```python
from build123d import *

# Parameters (mm, degrees)
SKETCH1_W           = 129
SKETCH1_H           = 74
BOSS_EXTRUDE1_DEPTH = 39
SKETCH2_R           = 1.5
CUT_EXTRUDE1_DEPTH  = 10
SKETCH4_W           = 129
SKETCH4_H           = 24
CUT_EXTRUDE3_DEPTH  = 100


with BuildPart() as part:
    # Sketch1 → Boss-Extrude1 (new body)
    with BuildSketch(Plane.XY):
        with Locations((64.5, 37)):
            Rectangle(SKETCH1_W, SKETCH1_H)
    extrude(amount=-BOSS_EXTRUDE1_DEPTH)

    # Sketch2 → Cut-Extrude1 (cut)
    with BuildSketch(Plane(origin=(0, 0, -39), x_dir=(-1, 0, 0), z_dir=(0, 0, -1))):
        with Locations((-50.3, 37)):
            Circle(SKETCH2_R)
        with Locations((-50.3, 55.35)):
            Circle(SKETCH2_R)
        with Locations((-50.3, 18.65)):
            Circle(SKETCH2_R)
        with Locations((-20.3, 55.35)):
            Circle(SKETCH2_R)
        with Locations((-20.3, 37)):
            Circle(SKETCH2_R)
        with Locations((-20.3, 18.65)):
            Circle(SKETCH2_R)
        with Locations((-112.7, 37)):
            Circle(SKETCH2_R)
        with Locations((-112.7, 53)):
            Circle(SKETCH2_R)
        with Locations((-110.1, 58.75)):
            Circle(SKETCH2_R)
        with Locations((-110.1, 46.75)):
            Circle(SKETCH2_R)
        with Locations((-110.1, 15.25)):
            Circle(SKETCH2_R)
        with Locations((-110.1, 27.25)):
            Circle(SKETCH2_R)
    extrude(amount=-CUT_EXTRUDE1_DEPTH, mode=Mode.SUBTRACT)

    # Cavity1: read off the stored shape, not the designer's step
    # Cavity1: loft between two sections, ruled curve by curve
    cavity1_from = [
        Edge.make_line((125.249, 3.561625, 0), (125.249, 70.427375, 0)),
        Edge.make_line((3.746, 3.561625, 0), (125.249, 3.561625, 0)),
        Edge.make_line((3.746, 70.427375, 0), (3.746, 3.561625, 0)),
        Edge.make_line((125.249, 70.427375, 0), (3.746, 70.427375, 0)),
    ]
    cavity1_to = [
        Edge.make_line((124.330201477, 4.483173045, -35.035), (124.330201477, 69.505826955, -35.035)),
        Edge.make_line((4.664798523, 4.483173045, -35.035), (124.330201477, 4.483173045, -35.035)),
        Edge.make_line((4.664798523, 69.505826955, -35.035), (4.664798523, 4.483173045, -35.035)),
        Edge.make_line((124.330201477, 69.505826955, -35.035), (4.664798523, 69.505826955, -35.035)),
    ]
    cavity1 = Solid(Shell([*[Face.make_surface_from_curves(cavity1_from[k], cavity1_to[k]) for k in range(4)], Face(Wire(cavity1_from)), Face(Wire(cavity1_to))]))
    add(cavity1, mode=Mode.SUBTRACT)

    # Sketch4 → Cut-Extrude3 (cut)
    with BuildSketch(Plane(origin=(0, 74, 0), x_dir=(1, 0, 0), z_dir=(0, 1, 0))):
        with Locations((64.5, 12)):
            Rectangle(SKETCH4_W, SKETCH4_H)
    extrude(amount=-CUT_EXTRUDE3_DEPTH, mode=Mode.SUBTRACT)


solid = part.part
```
Here's how the part is built. I have some questions about the finished solid (model axes, mm). A direction names the side the tool comes from. Give positions to 0.01 mm unless a question says otherwise; leave off trailing zeros. Answer as a JSON object with one key per item and string values. Group by question number.
Item 1: If we section it at A-A on y = 37: Give the number of separate pieces and of enclosed holes in the cut face, and give its area (3 significant figures).
Item 2: Please list where these lines run through material, in increasing order: probe 1 along Y at (x, z) = (110.1, -37.1); probe 2 along Y at (x, z) = (20.3, -37); probe 3 along Y at (x, z) = (29, -34).
Item 3: For P1, Ø1, axis at x = 89.5, y = 57, coming from the +Z side (3 decimals); P2, Ø2.5, axis at x = 110.1, y = 58.75, coming from the +Z side; P3, Ø5, axis at y = 45, z = -35, coming from the -X side, each with a flat end and sliding along its axis, tell me the tip position at first contact or that it passes through.
Item 4: If we mould it in two halves opening along X, with no side actions, what happens to faces 1 (the flat face through (0, 36, -31)), 2 (the flat face through (64, 70, -24)), 3 (the cylindrical face through (109.294, 60.015, -37.045))? For each: pulls with the +X half, pulls with the -X half, needs draft (parallel to the pull), parting line crosses it, or undercut.
Item 5: Which directions (+Z, -Z, +X, -X, +Y, -Y) give clear straight access to the entire face, cutting with the end or side of a thin tool? Please do faces 4 (the cylindrical face through (51.5, 36.1, -37)), 5 (the flat face through (64, 37, -35.035)).
Result set:
{
 "1": {"separate pieces": "4", "enclosed holes": "0", "area": "576 mm²"},
 "2": {"probe 1": "0 to 13.75, 16.75 to 25.75, 28.75 to 45.25, 48.25 to 57.25, 60.25 to 74", "probe 2": "0 to 17.15, 20.15 to 35.5, 38.5 to 53.85, 56.85 to 74", "probe 3": "0 to 4.46, 69.53 to 74"},
 "3": {"P1": "z = -35.035", "P2": "through", "P3": "x = 0"},
 "4": {"face 1": "pulls with the -X half", "face 2": "needs draft", "face 3": "undercut"},
 "5": {"face 4": "+Z, -Z", "face 5": "+Z"}
}
